Here's the drawing with two shaded views (mm, measured from the low corner). I have some questions. Round coordinates to 2 decimals unless told otherwise and drop trailing zeros. Loops run counter-clockwise (first coordinate to the right, second up) from the corner with the lowest first, then second, coordinate; pieces in that order, holes last.
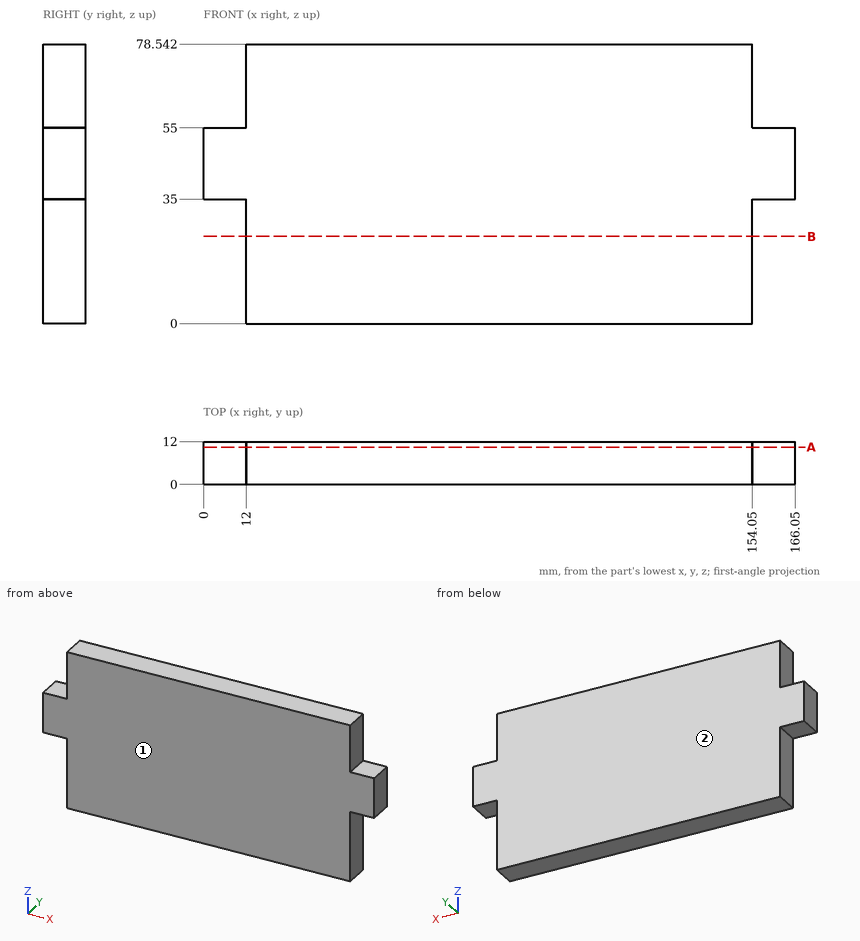
(1) If we mould it in two halves opening along Y, with no side actions, what happens to the marked faces 1 and 2? For each: released by +Y, released by -Y, zero draft, split by the parting line, or undercut.
Worked answers:
face 1: released by -Y
face 2: released by +Y
(2) If we section it at B-B, the plane z = 24.5: List the corners of the cut face in (x, y) for me.
Worked answers:
outline: (12, 0) - (154.05, 0) - (154.05, 12) - (12, 12) - close
(3) If we section it at A-A, the plane y = 10.5: List the corners of the cut face in (x, z) for me, then the cut area to 3 significant figures.
Worked answers:
outline: (0, 35) - (12, 35) - (12, 0) - (154.05, 0) - (154.05, 35) - (166.05, 35) - (166.05, 55) - (154.05, 55) - (154.05, 78.54) - (12, 78.54) - (12, 55) - (0, 55) - close
area: 11,600 mm2
(4) If I drill on line 1 (X direction, y = 2, z = 19.5), over which ranges is the centre line in solid material (lowest first)?
Worked answers:
line 1: x = 12 to 154.05
(5) Will these pins go through, and if not, where does the flat tip stop? P1, Ø6, axis at y = 6, z = 15, coming from the +X side; P2, Ø3.5, axis at y = 3.5, z = 71.5, coming from the -X side; P3, Ø3.5, axis at x = 160.5, y = 6.5, coming from the -Z side.
Worked answers:
P1: stops at x = 154.05
P2: stops at x = 12
P3: stops at z = 35
